```python
from build123d import *

# Parameters (mm, degrees)
F0_W     = 56.436695
F0_H     = 40.230245
F1_DEPTH = 25
F2_R     = 61.740337
F3_DEPTH = 64.786173


with BuildPart() as f1:
    # F0 (on Front) → F1 (new body)
    with BuildSketch(Plane.XZ):
        with Locations((1.673823, -6.281949)):
            Rectangle(F0_W, F0_H)
    extrude(amount=F1_DEPTH)

    # F2 (on Front) → F3 (join)
    with BuildSketch(Plane.XZ):
        Circle(F2_R)
    extrude(amount=-F3_DEPTH)


solid = f1.part
```
CAD build for the part. Positions are in the model's coordinates, mm. A direction names the side the tool comes from. Coordinates: 2 decimals unless noted, no trailing zeros. Write each loop counter-clockwise with the first axis right and the second up, starting at its lowest first coordinate (ties: lowest second). Pieces come first, ordered by that corner, then holes. Notation, with made-up numbers: (7.25, 51.5) -> (45.25, 51.5) arc R20 ccw to (45.25, 67.5) -> close; hole circle Ø3 at (9, 62.5). An arc over 180 degrees is marked (long way). Use CSV: the item, a comma, the result in double quotes. Start each with the question number.
Item 1: Two-plate mould, pull along X, no slides. Class faces 1 (the cylindrical face through (-13.384, 31.94, -60.272)), 2 (the flat face through (1, -12, 13.833)), 3 (the flat face through (29.892, -12, -7)), 4 (the flat face through (-26.545, -12, -7)): +X half, -X half, draft (parallel to the pull), parting line (faces both ways), or undercut.
Item 2: Band-saw the part on B-B, the plane x = 0. Write the cut outline in (y, z).
Item 3: Band-saw the part on D-D, the plane y = 55.5. Write the cut outline in (x, z), plus the area to 3 significant figures.
Item 4: Band-saw the part on C-C, the plane y = -3.5. Write the cut outline in (x, z).
Item 5: Band-saw the part on A-A, the plane z = 0. Write the cut outline in (x, y).
Item 6: Tool access for faces 5 (the flat face through (1, -12, -26.397)), 6 (the flat face through (1, -25, -6)): list every direction of +Z, -Z, +X, -X, +Y, -Y with a clear straight run to the whole face (end or side of a thin tool).
Item 7: Drop flat-ended pins along their axis: P1, Ø10, axis at x = 35.5, y = 33, coming from the +Z side; P2, Ø1.5, axis at y = 29.5, z = -1, coming from the -X side; P3, Ø10, axis at x = 25.5, y = 14.5, coming from the -Z side. Give the stop position or say it passes through.
Item 8: Wall check: probe 1 along Y at (x, z) = (11, 43); probe 2 along X at (y, z) = (-11.5, -1); probe 3 along Z at (x, y) = (-7, -11). Give the ranges that are in metal, low to high.
Response values:
1,face 1,"parting line"
1,face 2,"draft"
1,face 3,"+X half"
1,face 4,"-X half"
2,outline,"(-25, -26.4) -> (0, -26.4) -> (0, -61.74) -> (64.79, -61.74) -> (64.79, 61.74) -> (0, 61.74) -> (0, 13.83) -> (-25, 13.83) -> close"
3,outline,"circle Ø123.48 at (0, 0)"
3,area,"12,000 mm2"
4,outline,"(-26.54, -26.4) -> (29.89, -26.4) -> (29.89, 13.83) -> (-26.54, 13.83) -> close"
5,outline,"(-61.74, 0) -> (-26.54, 0) -> (-26.54, -25) -> (29.89, -25) -> (29.89, 0) -> (61.74, 0) -> (61.74, 64.79) -> (-61.74, 64.79) -> close"
6,face 5,"-Z, +X, -X, -Y"
6,face 6,"+Z, -Z, +X, -X, -Y"
7,P1,"stops at z = 53.68"
7,P2,"stops at x = -61.74"
7,P3,"stops at z = -58.24"
8,probe 1,"y = 0 to 64.79"
8,probe 2,"x = -26.54 to 29.89"
8,probe 3,"z = -26.4 to 13.83"
